Can you work these out from the drawing? Everything is in mm from the part's minimum corner. A direction names the side the tool comes from. Round coordinates to 2 decimals unless told otherwise and drop trailing zeros. Write each loop counter-clockwise with the first axis right and the second up, starting at its lowest first coordinate (ties: lowest second). Pieces come first, ordered by that corner, then holes. Notation, with made-up numbers: (19, 52) - (40, 52) arc R24 ccw to (40, 69) - close; hole circle Ø4 at (-38, 70.25). An arc over 180 degrees is marked (long way). One line per item, written item: value. Start each with the question number.
Item 1: For the marked faces 1 and 2, which set-ups out of +Z, -Z, +X, -X, +Y, -Y let a thin tool reach every point of the face, with its end or its side?
Item 2: Thinking about a two-plate mould opening in X: for the marked faces 3, 4 and 5, which applies, released by +X, released by -X, zero draft, split by the parting line, or undercut?
Item 3: Imagine slicing it at A-A, the plane y = 15.5. Please give me the cut outline in (x, z).
Item 4: If I drill on line 1 (Y direction, x = 5.5, z = 9.75); line 2 (X direction, y = 17.5, z = 6); line 3 (Z direction, x = 60.5, y = 15.5), over which ranges is the centre line in solid material (lowest first)?
Item 5: Imagine slicing it at C-C, the plane x = 64. Please give me the cut outline in (y, z).
Item 6: Imagine slicing it at B-B, the plane z = 11.25. Please give me the cut outline in (x, y).
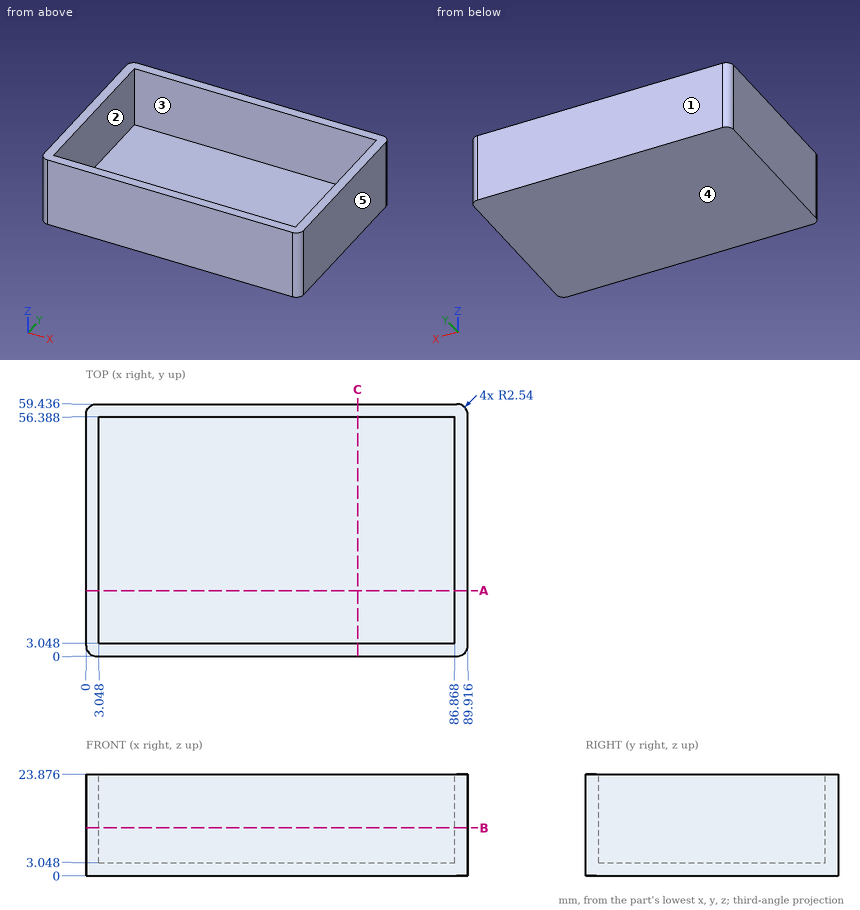
Values follow:
1. face 1: +Z, -Z, +X, -X, +Y
1. face 2: +Z
2. face 3: undercut
2. face 4: zero draft
2. face 5: released by +X
3. outline: (0, 0) - (89.92, 0) - (89.92, 23.88) - (86.87, 23.88) - (86.87, 3.05) - (3.05, 3.05) - (3.05, 23.88) - (0, 23.88) - close
4. line 1: y = 0 to 3.05, 56.39 to 59.44
4. line 2: x = 0 to 3.05, 86.87 to 89.92
4. line 3: z = 0 to 3.05
5. outline: (0, 0) - (59.44, 0) - (59.44, 23.88) - (56.39, 23.88) - (56.39, 3.05) - (3.05, 3.05) - (3.05, 23.88) - (0, 23.88) - close
6. outline: (0, 2.54) arc R2.54 ccw to (2.54, 0) - (87.38, 0) arc R2.54 ccw to (89.92, 2.54) - (89.92, 56.9) arc R2.54 ccw to (87.38, 59.44) - (2.54, 59.44) arc R2.54 ccw to (0, 56.9) - close; hole (3.05, 3.05) - (86.87, 3.05) - (86.87, 56.39) - (3.05, 56.39) - close
